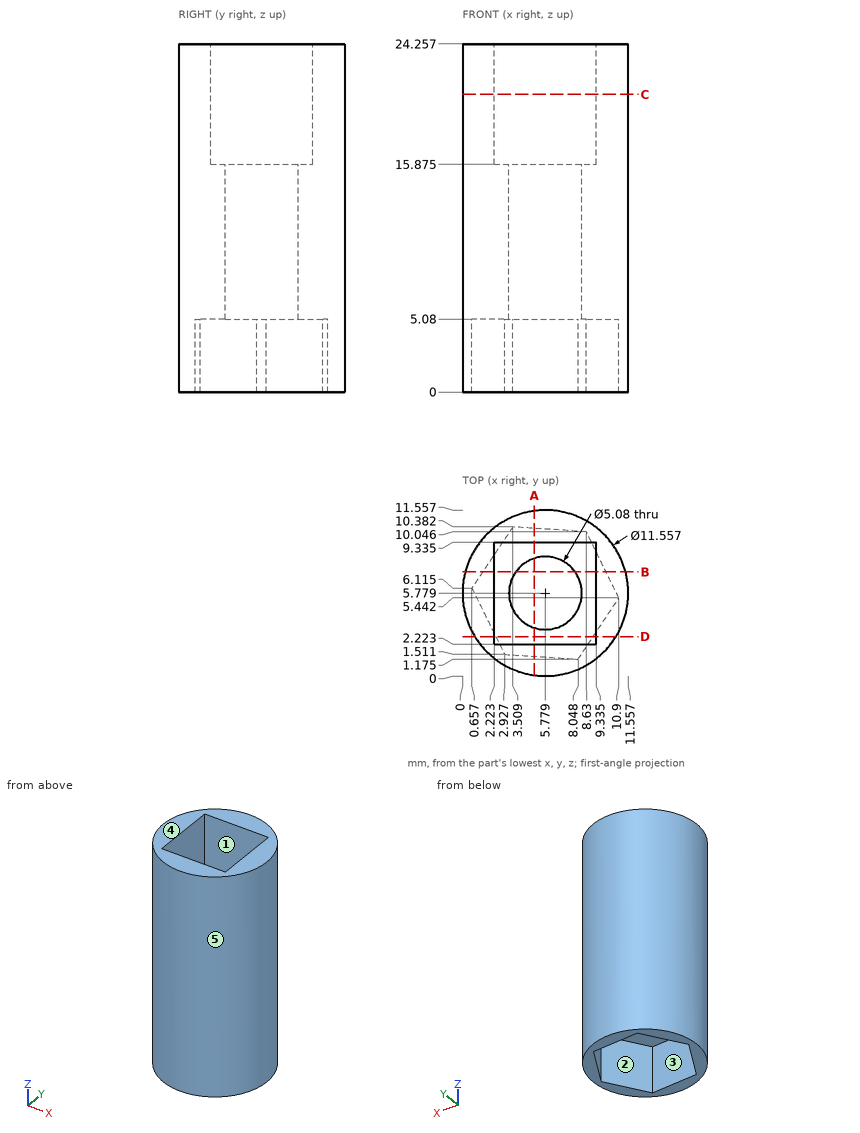
Drawing for the job (mm, zero at the part's lowest x, y, z). A direction names the side the tool comes from. Give positions to 0.01 mm unless a question says otherwise; leave off trailing zeros. Order: outer loops, then holes, each group sorted by start corner. A loop starts at its lowest first (then second) coordinate and runs counter-clockwise, first axis right, second up. Notation, with made-up numbers: (72.25, 48.5) - (85.25, 48.5) arc R28 ccw to (85.25, 82.5) - close; hole circle Ø11 at (34.5, -22.75). An arc over 180 degrees is marked (long way). Use one line per item in the form item = value.
Item 1: Slice it at A-A on x = 5. Give the cut face in (y, z) (1 decimal), and give its area (3 significant figures).
Solution:
outline = (0.1, 0) - (1.4, 0) - (1.4, 5.1) - (3.4, 5.1) - (3.4, 15.9) - (2.2, 15.9) - (2.2, 24.3) - (0.1, 24.3) - close; (8.2, 5.1) - (10.3, 5.1) - (10.3, 0) - (11.5, 0) - (11.5, 24.3) - (9.3, 24.3) - (9.3, 15.9) - (8.2, 15.9) - close
area = 121 mm2
Item 2: Slice it at B-B on y = 7.25. Give the cut face in (x, z) (1 decimal), and give its area (3 significant figures).
Solution:
outline = (0.2, 0) - (1.4, 0) - (1.4, 5.1) - (3.7, 5.1) - (3.7, 15.9) - (2.2, 15.9) - (2.2, 24.3) - (0.2, 24.3) - close; (7.8, 5.1) - (10, 5.1) - (10, 0) - (11.4, 0) - (11.4, 24.3) - (9.3, 24.3) - (9.3, 15.9) - (7.8, 15.9) - close
area = 123 mm2
Item 3: Two-plate mould, pull along Y, no slides. Class the marked faces 3, 4 and 5: released by +Y, released by -Y, zero draft, split by the parting line, or undercut.
Solution:
face_3 = undercut
face_4 = zero draft
face_5 = split by the parting line
Item 4: Pin check, flat tips, straight feed: pin 1 Ø1.5 at (y, z) = (4, 21) entering from -X; pin 2 Ø3 at (y, z) = (10, 11.5) entering from +X (1 decimal); pin 3 Ø2 at (x, y) = (3, 6) entering from -Z; pin 4 Ø3 at (x, y) = (5.78, 5.78) entering from -Z. Stop position of each tip, or through.
Solution:
pin_1 = 0.09
pin_2 = 10.9
pin_3 = 5.08
pin_4 = through
Item 5: Slice it at C-C on z = 20.75. Give the cut face in (x, y) (1 decimal).
Solution:
outline = circle Ø11.6 at (5.8, 5.8); hole (2.2, 2.2) - (9.3, 2.2) - (9.3, 9.3) - (2.2, 9.3) - close
Item 6: Which spindle directions (+Z, -Z, +X, -X, +Y, -Y) get a long thin tool onto all of the face, cutting with end or side? Do the marked faces 1 and 2. Say none if no direction does.
Solution:
face_1 = +Z
face_2 = -Z
Item 7: Slice it at D-D on y = 2.75. Give the cut face in (x, z) (1 decimal), and give its area (3 significant figures).
Solution:
outline = (0.9, 0) - (2.3, 0) - (2.3, 5.1) - (9.1, 5.1) - (9.1, 0) - (10.7, 0) - (10.7, 24.3) - (9.3, 24.3) - (9.3, 15.9) - (2.2, 15.9) - (2.2, 24.3) - (0.9, 24.3) - close
area = 145 mm2
Item 8: Probe probe 1 along Y at (x, z) = (6, 19) (1 decimal); probe 2 along Z at (x, y) = (2.75, 2.75) (1 decimal); probe 3 along X at (y, z) = (6.25, 6.5) (1 decimal). List the from-to ranges inside material, lowest first. Write a range as from..to.
Solution:
probe_1 = 0..2.2, 9.3..11.6
probe_2 = 5.1..15.9
probe_3 = 0..3.3, 8.3..11.5
